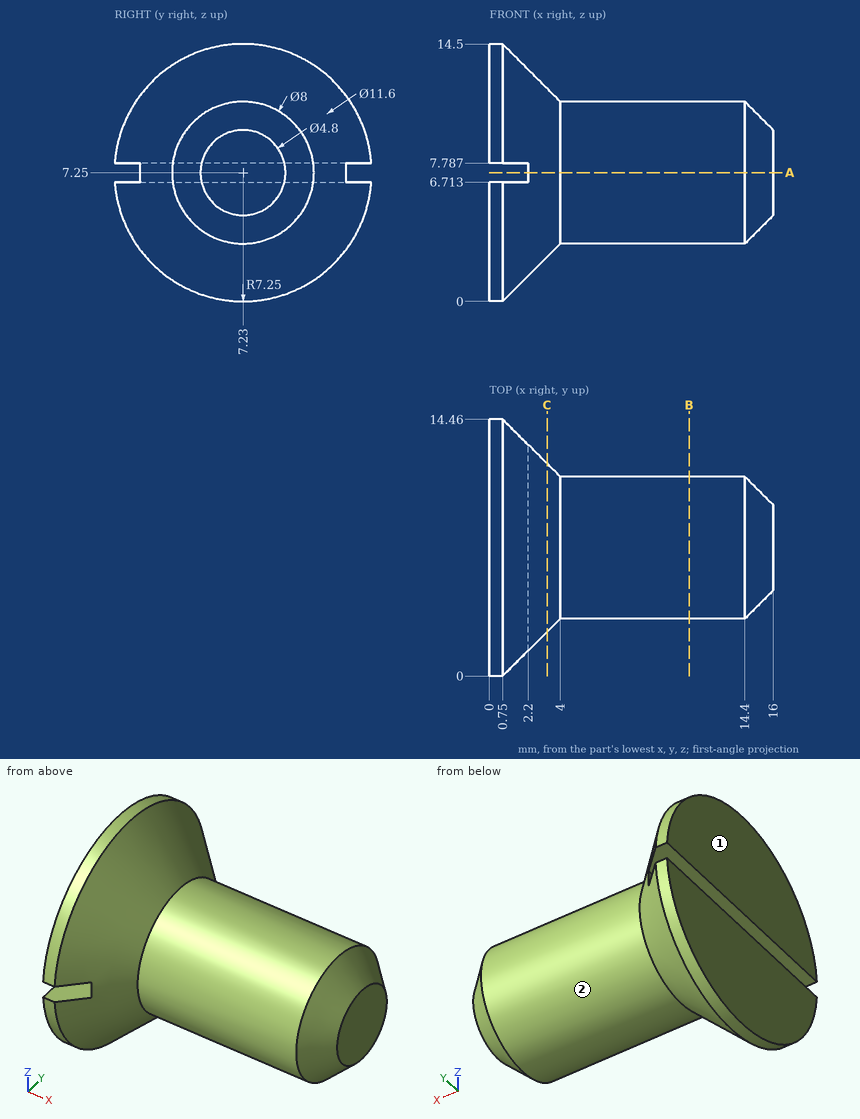
Here's the drawing with two shaded views (mm, measured from the low corner). I have some questions. A direction names the side the tool comes from. Coordinates: 2 decimals unless noted, no trailing zeros. Loops run counter-clockwise (first coordinate to the right, second up) from the corner with the lowest first, then second, coordinate; pieces in that order, holes last. Notation, with made-up numbers: (-16, 33) -> (-5, 33) arc R23 cw to (-5, 72) -> close; hole circle Ø3 at (48.25, 33). An arc over 180 degrees is marked (long way). Use one line per item in the form item = value. Start each with the question number.
(1) Will these pins go through, and if not, where does the flat tip stop? pin 1 (1.5 mm diameter, centred on x = 13, z = 6.5, fed in from -Y); pin 2 (5 mm diameter, centred on x = 10.5, y = 8, fed in from +Z); pin 3 (8 mm diameter, centred on x = 3.5, z = 10, fed in from +Y); pin 4 (0.7 mm diameter, centred on x = 1.5, y = 6.5, fed in from +Z).
(2) If we section it at B-B (x = 11.25): Please give me the cut outline in (y, z).
(3) On a 3-axis mill with a long thin cutter (end or side, diameter ignored), from which of +Z, -Z, +X, -X, +Y, -Y can I reach the whole of each face in a straight line? I mean the marked faces 1 and 2. Say none if no direction works.
(4) If we section it at C-C (x = 3.25): Please give me the cut outline in (y, z), then the cut area to 3 significant figures.
(5) Please list where these lines run through material, in increasing order: line 1 along X through (y, z) = (8, 3.75) (1 decimal); line 2 along Z through (x, y) = (3.75, 10.25); line 3 along Z through (x, y) = (4.25, 9.5) (1 decimal).
(6) If we section it at A-A (z = 7.25): Please give me the cut outline in (x, y).
Verdict:
q1.pin_1 = 3.23
q1.pin_2 = 11.25
q1.pin_3 = 14.46
q1.pin_4 = 14.06
q2.outline = circle Ø8 at (7.23, 7.25)
q3.face_1 = +Z, -Z, -X, +Y, -Y
q3.face_2 = +X
q4.outline = circle Ø9.5 at (7.23, 7.25)
q4.area = 70.9 mm²
q5.line_1 = 0 to 14.8
q5.line_2 = 4.26 to 10.24
q5.line_3 = 4 to 10.5
q6.outline = (2.2, 1.43) -> (4, 3.23) -> (14.4, 3.23) -> (16, 4.83) -> (16, 9.63) -> (14.4, 11.23) -> (4, 11.23) -> (2.2, 13.03) -> close
